Build history of the part. All positions in model axes, mm. Face numbers are marked on the shaded views. A direction names the side the tool comes from. Round coordinates to 2 decimals unless told otherwise and drop trailing zeros. Order: outer loops, then holes, each group sorted by start corner. A loop starts at its lowest first (then second) coordinate and runs counter-clockwise, first axis right, second up. Notation, with made-up numbers: (86, 60) -> (118, 60) arc R10 cw to (118, 73) -> close; hole circle Ø7 at (-19.5, 22.25). An arc over 180 degrees is marked (long way). Use a Markdown table: item, result. Add a question column.
Item 1: Pin check, flat tips, straight feed: pin 1 (3 mm diameter, centred on y = -8.5, z = 12, fed in from +X); pin 2 (10.5 mm diameter, centred on x = -2, y = -2, fed in from -Z) (3 decimals); pin 3 (8 mm diameter, centred on y = 8.5, z = 19.5, fed in from +X). Stop position of each tip, or through.
Item 2: 3-axis set-ups, long thin cutter, end or side, ignore diameter. For the marked faces 4 and 5: which of +Z, -Z, +X, -X, +Y, -Y reach the whole face in a straight line?
Item 3: Two-plate mould, pull along X, no slides. Class the marked faces 1, 2 and 3: released by +X, released by -X, zero draft, split by the parting line, or undercut.
Item 4: Slice it at A-A, the plane y = 0. Give the cut face in (x, z), plus the area to 3 significant figures.
Item 5: Probe L1, parallel to Y at x = 0, z = 0.2; L2, parallel to Y at x = 0, z = 1.8; L3, parallel to Z at x = -6, y = -8.75. List the from-to ranges inside material, lowest first.
Item 6: Slice it at D-D, the plane y = -9.5. Give the cut face in (x, z), plus the area to 3 significant figures.
Item 7: Slice it at C-C, the plane z = 9. Give the cut face in (x, y), plus the area to 3 significant figures.
from build123d import *

# Parameters (mm, degrees)
SKETCH1_R               = 12.7
BOSS_EXTRUDE1_DEPTH     = 25.4
SKETCH2_R               = 10.4
CUT_EXTRUDE1_DEPTH      = 5.5
CUT_EXTRUDE2_START      = -1
SKETCH3_R               = 11.75
CUT_EXTRUDE2_DEPTH      = 1.8
F_1_4_28_TAPPED_HOLE1_D = 5.4102


with BuildPart() as part:
    # Sketch1 → Boss-Extrude1 (new body)
    with BuildSketch(Plane.XY):
        Circle(SKETCH1_R)
    extrude(amount=BOSS_EXTRUDE1_DEPTH)

    # Sketch2 → Cut-Extrude1 (cut)
    with BuildSketch(Plane(origin=(0, 0, 0), x_dir=(-1, 0, 0), z_dir=(0, 0, -1))):
        Circle(SKETCH2_R)
    extrude(amount=-CUT_EXTRUDE1_DEPTH, mode=Mode.SUBTRACT)

    # Sketch3 → Cut-Extrude2 (cut)
    with BuildSketch(Plane(origin=(0, 0, 0), x_dir=(-1, 0, 0), z_dir=(0, 0, -1)).offset(CUT_EXTRUDE2_START)):
        Circle(SKETCH3_R)
    extrude(amount=-CUT_EXTRUDE2_DEPTH, mode=Mode.SUBTRACT)

    # 1/4-28 Tapped Hole1 (through all)
    with Locations(Plane.XY.offset(25.4)):
        with Locations((0, 0)):
            Hole(F_1_4_28_TAPPED_HOLE1_D / 2)

    # Sketch10 → Cut-Revolve1 (revolve, cut)
    with BuildSketch(Plane(origin=(0, 0, 0), x_dir=(1, 0, 0), z_dir=(0, 1, 0))):
        Polygon((0, -25.402256059), (8.654624222, -5.5), (0, -5.5), align=None)
    revolve(axis=Axis((0, 0, 29.736025406), (0, 0, -1)), mode=Mode.SUBTRACT)


solid = part.part
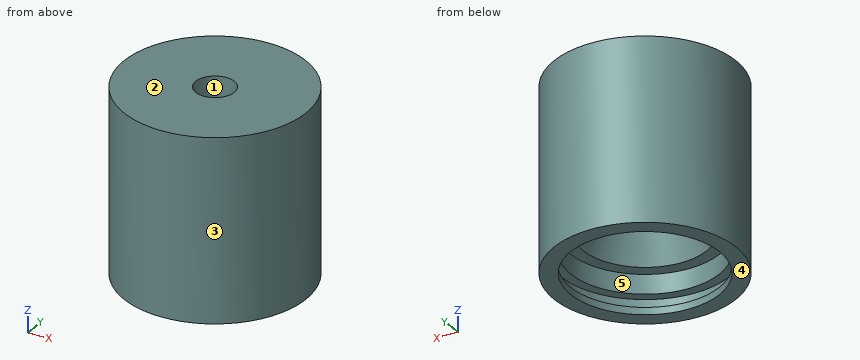
Check sheet entries:
| question | item | result |
|---|---|---|
| 1 | pin 1 | x = 10.6 |
| 1 | pin 2 | z = 6.825 |
| 1 | pin 3 | x = 11.88 |
| 2 | face 4 | -Z, +X, -X, +Y, -Y |
| 2 | face 5 | -Z |
| 3 | face 1 | undercut |
| 3 | face 2 | zero draft |
| 3 | face 3 | split by the parting line |
| 4 | outline | (-12.7, 0) -> (-10.4, 0) -> (-10.4, 1) -> (-11.75, 1) -> (-11.75, 2.8) -> (-10.4, 2.8) -> (-10.4, 5.5) -> (-8.65, 5.5) -> (-2.71, 19.18) -> (-2.71, 25.4) -> (-12.7, 25.4) -> close; (2.71, 19.18) -> (8.65, 5.5) -> (10.4, 5.5) -> (10.4, 2.8) -> (11.75, 2.8) -> (11.75, 1) -> (10.4, 1) -> (10.4, 0) -> (12.7, 0) -> (12.7, 25.4) -> (2.71, 25.4) -> close |
| 4 | area | 337 mm2 |
| 5 | L1 | -12.7 to -10.4, 10.4 to 12.7 |
| 5 | L2 | -12.7 to -11.75, 11.75 to 12.7 |
| 5 | L3 | 0 to 1, 2.8 to 25.4 |
| 6 | outline | (-8.43, 0) -> (-4.23, 0) -> (-4.23, 1) -> (-6.91, 1) -> (-6.91, 2.8) -> (-4.23, 2.8) -> (-4.23, 5.5) -> (4.23, 5.5) -> (4.23, 2.8) -> (6.91, 2.8) -> (6.91, 1) -> (4.23, 1) -> (4.23, 0) -> (8.43, 0) -> (8.43, 25.4) -> (-8.43, 25.4) -> close |
| 6 | area | 372 mm2 |
| 7 | outline | circle Ø25.4 at (0, 0); hole circle Ø14.27 at (0, 0) |
| 7 | area | 347 mm2 |
